from build123d import *

# Parameters (mm, degrees)
BOSS_EXTRUDE1_DEPTH = 3.048
SKETCH2_R           = 1.355900406
CUT_EXTRUDE1_DEPTH  = 4.048
SKETCH3_R           = 1.524
CUT_EXTRUDE2_DEPTH  = 4.048
CUT_EXTRUDE3_DEPTH  = 4.048
BOSS_EXTRUDE2_DEPTH = 3.048
SKETCH5_W           = 11.049
SKETCH5_H           = 14.8839
SKETCH5_W_2         = 76.4276
SKETCH5_H_2         = 52.6961
SKETCH5_H_3         = 14.1902
CUT_EXTRUDE4_DEPTH  = 4.048


with BuildPart() as part:
    # Sketch1 → Boss-Extrude1 (new body)
    with BuildSketch(Plane.XY):
        with BuildLine():
            Line((-309.8086, 128.8851), (-305.87795, 128.8851))
            Line((-305.87795, 128.8851), (-301.9473, 132.81575))
            Line((-301.9473, 132.81575), (-301.9473, 150.9704))
            ThreePointArc((-301.9473, 150.9704), (-303.063223164, 153.664476836), (-305.7573, 154.7804))
            Line((-305.7573, 154.7804), (-397.247125, 154.7804))
            ThreePointArc((-397.247125, 154.7804), (-399.946077222, 153.659592612), (-401.0571, 150.956597849))
            Line((-401.0571, 150.956597849), (-401.0571, 148.341))
            Line((-401.0571, 148.341), (-399.1521, 148.341))
            Line((-399.1521, 148.341), (-399.1521, 95.6449))
            Line((-399.1521, 95.6449), (-401.0571, 95.6449))
            Line((-401.0571, 95.6449), (-401.0571, 91.659304166))
            ThreePointArc((-401.0571, 91.659304166), (-399.951018769, 88.947400452), (-397.2472, 87.8217))
            Line((-397.2472, 87.8217), (-378.5565, 87.8217))
            Line((-378.5565, 87.8217), (-368.3165, 91.1883))
            Line((-368.3165, 91.1883), (-315.9973, 91.1883))
            Line((-315.9973, 91.1883), (-305.7573, 87.8217))
            ThreePointArc((-305.7573, 87.8217), (-303.063223164, 88.937623164), (-301.9473, 91.6317))
            Line((-301.9473, 91.6317), (-301.9473, 111.74645))
            Line((-301.9473, 111.74645), (-305.87795, 115.6771))
            Line((-305.87795, 115.6771), (-309.8086, 115.6771))
            Line((-309.8086, 115.6771), (-314.0123, 115.6771))
            Line((-314.0123, 115.6771), (-314.0123, 128.8851))
            Line((-314.0123, 128.8851), (-309.8086, 128.8851))
        make_face()
        Polygon((-395.3675, 92.9525), (-395.3675, 149.2432), (-309.8086, 149.2432), (-309.8086, 132.81575), (-318.2033, 132.81575), (-318.2033, 111.74645), (-309.8086, 111.74645), (-309.8086, 92.9525), align=None, mode=Mode.SUBTRACT)
    extrude(amount=BOSS_EXTRUDE1_DEPTH)

    # Sketch2 → Cut-Extrude1 (cut, through all)
    with BuildSketch(Plane(origin=(0, 0, 0), x_dir=(-1, 0, 0), z_dir=(0, 0, -1))):
        with Locations((305.7573, 150.9704)):
            Circle(SKETCH2_R)
        with Locations((397.247125, 150.9704)):
            Circle(SKETCH2_R)
        with Locations((397.2472, 91.6317)):
            Circle(SKETCH2_R)
        with Locations((305.7573, 91.6317)):
            Circle(SKETCH2_R)
    extrude(amount=-CUT_EXTRUDE1_DEPTH, mode=Mode.SUBTRACT)

    # Sketch3 → Cut-Extrude2 (cut, through all)
    with BuildSketch(Plane(origin=(0, 0, 0), x_dir=(-1, 0, 0), z_dir=(0, 0, -1))):
        with Locations((305.7573, 150.9704)):
            Circle(SKETCH3_R)
        with Locations((397.247125, 150.9704)):
            Circle(SKETCH3_R)
        with Locations((397.2472, 91.6317)):
            Circle(SKETCH3_R)
        with Locations((305.7573, 91.6317)):
            Circle(SKETCH3_R)
    extrude(amount=-CUT_EXTRUDE2_DEPTH, mode=Mode.SUBTRACT)

    # Sketch4 → Cut-Extrude3 (cut, through all)
    with BuildSketch(Plane.XY.offset(3.048)):
        Polygon((-301.9473, 133.57775), (-305.87795, 129.6471), (-314.0123, 129.6471), (-314.0123, 113.6451), (-305.87795, 113.6451), (-301.9473, 109.71445), align=None)
    extrude(amount=-CUT_EXTRUDE3_DEPTH, mode=Mode.SUBTRACT)

    # Sketch4_4 → Boss-Extrude2 (add)
    with BuildSketch(Plane.XY.offset(3.048)):
        Polygon((-318.2033, 111.74645), (-318.2033, 132.81575), (-309.8086, 132.81575), (-309.8086, 149.2432), (-395.3675, 149.2432), (-395.3675, 92.9525), (-309.8086, 92.9525), (-309.8086, 111.74645), align=None)
    extrude(amount=-BOSS_EXTRUDE2_DEPTH)

    # Sketch5 → Cut-Extrude4 (cut, through all)
    with BuildSketch(Plane.XY.offset(3.048)):
        with Locations((-312.2978, 140.89905)):
            Rectangle(SKETCH5_W, SKETCH5_H)
        with Locations((-356.0361, 121.99295)):
            Rectangle(SKETCH5_W_2, SKETCH5_H_2)
        with Locations((-312.2978, 102.74)):
            Rectangle(SKETCH5_W, SKETCH5_H_3)
    extrude(amount=-CUT_EXTRUDE4_DEPTH, mode=Mode.SUBTRACT)


solid = part.part
Work out the finished part from the listing and answer in its coordinate system (mm). A direction names the side the tool comes from. Round coordinates to 2 decimals unless told otherwise and drop trailing zeros. Loops run counter-clockwise (first coordinate to the right, second up) from the corner with the lowest first, then second, coordinate; pieces in that order, holes last. Notation, with made-up numbers: M 89.25,1 L 104.25,1 A23 ccw 104.25,32 Z; hole C -13,56 d10. An arc over 180 degrees is marked long. One line per question, with ' | ' between items. Start each with the question number.
(1) A cutting plane is placed at D-D on x = -313. Write down the section's boundary in (y, z), plus the area to 3 significant figures.
(2) Flat-ended cylindrical pins translate along their axes: pin 1 Ø0.6 at (x, z) = (-400.5, 1.5) entering from +Y; pin 2 Ø1.5 at (x, z) = (-311.5, 1) entering from -Y; pin 3 Ø0.9 at (x, z) = (-350, 1.5) entering from -Y. Find the tip coordinate at first contact, or state that the pin passes through.
(3) Find the intervals of material crossed by line 1 (Y direction, x = -325, z = 1.85); line 2 (Y direction, x = -308, z = 2.7); line 3 (X direction, y = 138, z = 1.1), in increasing order.
(4) A tool of negligible diameter and unlimited length cuts with its end or side. For faces 4 (the face through (-306.773, 103, 2)), 5 (the face through (-400, 95.645, 2)), 6 (the face through (-343, 91.188, 2)), from which of +Z, -Z, +X, -X, +Y, -Y can it reach the whole face along a straight path? Write none if from no direction.
(5) A cutting plane is placed at B-B on x = -381. Write down the section's boundary in (y, z), plus the area to 3 significant figures.
(6) For a pull along X with two mould halves and no side action, classify faces 1 (the face through (-398.655, 91.048, 1.503)), 2 (the face through (-301.947, 101, 2)), 3 (the face through (-400, 89, 2)) as released by +X, released by -X, zero draft, split by the parting line, or undercut.
(7) A cutting plane is placed at A-A on y = 105. Write down the section's boundary in (x, z), plus the area to 3 significant figures.
(8) A cutting plane is placed at C-C on z = 2.45. Give the number of separate pieces and of enclosed holes in the cut face, plus the area to 3 significant figures.
Geometry check:
1) outline: M 90.2,0 L 95.64,0 L 95.64,3.05 L 90.2,3.05 Z; M 109.84,0 L 113.65,0 L 113.65,3.05 L 109.84,3.05 Z; M 129.65,0 L 133.46,0 L 133.46,3.05 L 129.65,3.05 Z; M 148.34,0 L 154.78,0 L 154.78,3.05 L 148.34,3.05 Z | area: 59.4 mm²
2) pin 1: stops at y = 153.38 | pin 2: stops at y = 89.46 | pin 3: stops at y = 91.19
3) line 1: y = 91.19 to 95.64, 148.34 to 154.78 | line 2: y = 88.56 to 95.64, 109.84 to 113.65, 129.65 to 133.46, 148.34 to 154.78 | line 3: x = -399.15 to -394.25, -306.77 to -301.95
4) face 4: +Z, -Z | face 5: +Z, -Z, -X | face 6: +Z, -Z, -Y
5) outline: M 87.82,0 L 95.64,0 L 95.64,3.05 L 87.82,3.05 Z; M 148.34,0 L 154.78,0 L 154.78,3.05 L 148.34,3.05 Z | area: 43.5 mm²
6) face 1: undercut | face 2: released by +X | face 3: released by -X
7) outline: M -399.15,0 L -394.25,0 L -394.25,3.05 L -399.15,3.05 Z; M -306.77,0 L -301.95,0 L -301.95,3.05 L -306.77,3.05 Z | area: 29.7 mm²
8) separate pieces: 1 | enclosed holes: 5 | area: 1,730 mm²
